```python
from build123d import *

# Parameters (mm, degrees)
SKETCH1_R                 = 19.05
BOSS_EXTRUDE1_DEPTH       = 63.5
FILLET1_R                 = 3.81
SKETCH2_R                 = 3.81
BOSS_EXTRUDE2_DEPTH       = 2.54
F_8_32_TAPPED_HOLE1_D     = 3.4544
F_8_32_TAPPED_HOLE1_DEPTH = 12.53744
F_8_32_TAPPED_HOLE1_TIP   = 1.037806461
SKETCH6_W                 = 16.907326274
SKETCH6_H                 = 52.824444264


with BuildPart() as part:
    # Sketch1 → Boss-Extrude1 (new body)
    with BuildSketch(Plane(origin=(0, 0, 0), x_dir=(1, 0, 0), z_dir=(0, 1, 0))):
        Circle(SKETCH1_R)
    extrude(amount=BOSS_EXTRUDE1_DEPTH)

    # Fillet1
    fillet1_edges = [part.edges().sort_by_distance(p)[0] for p in [
        (-19.05, 0, 0),
        (-19.05, 63.5, 0),
    ]]
    fillet(fillet1_edges, radius=FILLET1_R)

    # Sketch2 → Boss-Extrude2 (add)
    with BuildSketch(Plane(origin=(0, 63.5, 0), x_dir=(1, 0, 0), z_dir=(0, 1, 0))):
        Circle(SKETCH2_R)
    extrude(amount=BOSS_EXTRUDE2_DEPTH)

    # #8-32 Tapped Hole1
    with Locations(Plane(origin=(0, 66.04, 0), x_dir=(1, 0, 0), z_dir=(0, 1, 0))):
        with Locations((0, 0)):
            Hole(F_8_32_TAPPED_HOLE1_D / 2, depth=F_8_32_TAPPED_HOLE1_DEPTH)
            with Locations((0, 0, -(F_8_32_TAPPED_HOLE1_DEPTH + F_8_32_TAPPED_HOLE1_TIP / 2))):  # 118° drill point
                Cone(0, F_8_32_TAPPED_HOLE1_D / 2, F_8_32_TAPPED_HOLE1_TIP, mode=Mode.SUBTRACT)

    # Sketch6 → Cut-Revolve1 (revolve, cut)
    with BuildSketch(Plane(origin=(0, 0, 0), x_dir=(0, 0, -1), z_dir=(1, 0, 0))):
        with Locations((8.453663137, 31.924965915)):
            Rectangle(SKETCH6_W, SKETCH6_H)
    revolve(axis=Axis((0, 5.512743783, 0), (0, 1, 0)), mode=Mode.SUBTRACT)


solid = part.part
```
Could you check a few things on this model? Use its own coordinates, in mm. A direction names the side the tool comes from. Round coordinates to 2 decimals unless told otherwise and drop trailing zeros. Loops run counter-clockwise (first coordinate to the right, second up) from the corner with the lowest first, then second, coordinate; pieces in that order, holes last. Notation, with made-up numbers: (36, 57) -> (83, 57) arc R22 cw to (83, 83) -> close; hole circle Ø10 at (86.5, 16.5). An arc over 180 degrees is marked (long way). Put each result on its own line as item: value.
Q1. Which directions (+Z, -Z, +X, -X, +Y, -Y) give clear straight access to the entire face, cutting with the end or side of a thin tool? Please do faces 1 (the flat face through (4, 58.337, 0)), 2 (the flat face through (0, 0, 0)), 3 (the cylindrical face through (-0.83, 64.75, 3.72)).
Checks:
face 1: none
face 2: +Z, -Z, +X, -X, -Y
face 3: +Y
Q2. I want a section at A-A on z = 0. Write out the boundary of the cut face in (x, y), and give its area (3 significant figures).
Checks:
outline: (-19.05, 3.81) arc R3.81 ccw to (-15.24, 0) -> (15.24, 0) arc R3.81 ccw to (19.05, 3.81) -> (19.05, 59.69) arc R3.81 ccw to (15.24, 63.5) -> (3.81, 63.5) -> (3.81, 66.04) -> (1.73, 66.04) -> (1.73, 58.34) -> (16.91, 58.34) -> (16.91, 5.51) -> (-16.91, 5.51) -> (-16.91, 58.34) -> (-1.73, 58.34) -> (-1.73, 66.04) -> (-3.81, 66.04) -> (-3.81, 63.5) -> (-15.24, 63.5) arc R3.81 ccw to (-19.05, 59.69) -> close
area: 613 mm2
Q3. For pin 1 Ø8 at (y, z) = (30.5, 9) entering from +X; pin 2 Ø3 at (x, z) = (13.5, -12) entering from -Y; pin 3 Ø1 at (x, y) = (-5, 32) entering from -Z, each with a flat end and sliding along its axis, tell me the tip position at first contact or that it passes through.
Checks:
pin 1: x = 18.38
pin 2: y = 0.24
pin 3: z = -18.51
Q4. I want a section at C-C on y = 57.5. Write out the boundary of the cut face in (x, z), and give its area (3 significant figures).
Checks:
outline: circle Ø38.1 at (0, 0); hole circle Ø33.81 at (0, 0)
area: 242 mm2
Q5. I want a section at B-B on x = 0. Write out the boundary of the cut face in (y, z), and give its area (3 significant figures).
Checks:
outline: (0, -15.24) arc R3.81 ccw to (3.81, -19.05) -> (59.69, -19.05) arc R3.81 ccw to (63.5, -15.24) -> (63.5, -3.81) -> (66.04, -3.81) -> (66.04, -1.73) -> (58.34, -1.73) -> (58.34, -16.91) -> (5.51, -16.91) -> (5.51, 16.91) -> (58.34, 16.91) -> (58.34, 1.73) -> (66.04, 1.73) -> (66.04, 3.81) -> (63.5, 3.81) -> (63.5, 15.24) arc R3.81 ccw to (59.69, 19.05) -> (3.81, 19.05) arc R3.81 ccw to (0, 15.24) -> close
area: 613 mm2
Q6. Thinking about a two-plate mould opening in Z: for faces 4 (the cylindrical face through (-15.12, 31.36, 11.59)), 5 (the flat face through (2, 66.04, 1)), 6 (the flat face through (0, 5.513, 0)), which applies, pulls with the +Z half, pulls with the -Z half, needs draft (parallel to the pull), parting line crosses it, or undercut?
Checks:
face 4: parting line crosses it
face 5: needs draft
face 6: undercut
Q7. Please list where these lines run through material, in increasing order: line 1 (Y direction, x = -14.5, z = -4); line 2 (Z direction, x = 0.5, y = 42); line 3 (Z direction, x = 0, y = 64). Write a range as from..to.
Checks:
line 1: 0..5.51, 58.34..63.5
line 2: -19.04..-16.9, 16.9..19.04
line 3: -3.81..-1.73, 1.73..3.81
